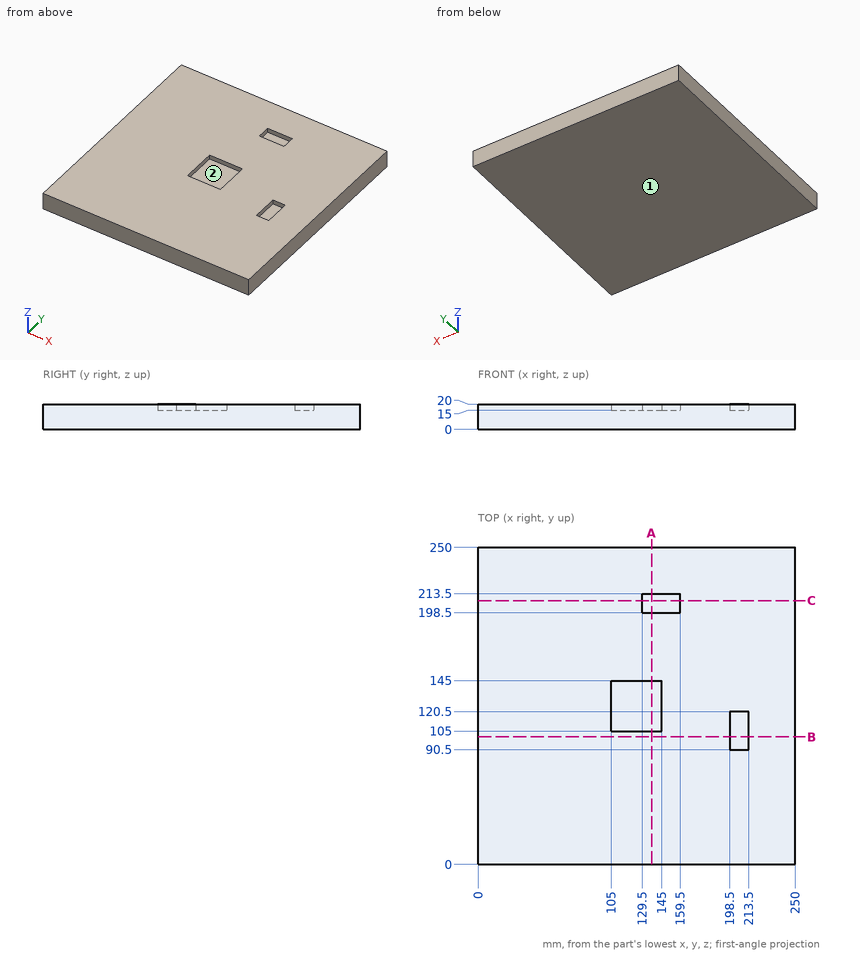
Part print with two shaded views. Sizes in mm from the minimum x, y, z corner. Round coordinates to 2 decimals unless told otherwise and drop trailing zeros. Order: outer loops, then holes, each group sorted by start corner. A loop starts at its lowest first (then second) coordinate and runs counter-clockwise, first axis right, second up. Notation, with made-up numbers: M 62.5,70 L 86.5,70 A16 cw 86.5,75 Z; hole C 69.5,15 d8. An arc over 180 degrees is marked long. Use CSV: the item, a comma, the result in double quotes. Start each with the question number.
(1) Mould opens along X. For the marked faces 1 and 2 say: +X half, -X half, draft (parallel to the pull), parting line (faces both ways), or undercut.
(2) Drill centre lines: probe 1 along Z at (x, y) = (141, 140); probe 2 along X at (y, z) = (125, 19). Where is each one in solid material? Low to high.
(3) Cut at A-A on x = 137. List the corners of the cut face in (y, z).
(4) Flat gauge pin, fed straight in: P1, Ø4.5, axis at x = 202.5, y = 99.5, coming from the +Z side. Where does the tip first touch, or does it go through?
(5) Cut at C-C on y = 208. List the corners of the cut face in (x, z), then the cut area to 3 significant figures.
(6) Cut at B-B on y = 100.5. List the corners of the cut face in (x, z), then the cut area to 4 significant figures.
Findings:
1,face 1,"draft"
1,face 2,"undercut"
2,probe 1,"z = 0 to 15"
2,probe 2,"x = 0 to 105, 145 to 250"
3,outline,"M 0,0 L 250,0 L 250,20 L 213.5,20 L 213.5,15 L 198.5,15 L 198.5,20 L 145,20 L 145,15 L 105,15 L 105,20 L 0,20 Z"
4,P1,"stops at z = 15"
5,outline,"M 0,0 L 250,0 L 250,20 L 159.5,20 L 159.5,15 L 129.5,15 L 129.5,20 L 0,20 Z"
5,area,"4,850 mm^2"
6,outline,"M 0,0 L 250,0 L 250,20 L 213.5,20 L 213.5,15 L 198.5,15 L 198.5,20 L 0,20 Z"
6,area,"4,925 mm^2"
